```python
from build123d import *

# Parameters (mm, degrees)
BOSS_EXTRUDE1_DEPTH = 5
SKETCH3_R           = 1.25
CUT_EXTRUDE1_DEPTH  = 215.675530355
CIRPATTERN2_COUNT   = 6
FILLET3_R           = 2.5
FILLET4_R           = 60


with BuildPart() as part:
    # Sketch1 → Boss-Extrude1 (new body)
    with BuildSketch(Plane(origin=(0, 0, 0), x_dir=(1, 0, 0), z_dir=(0, 1, 0))):
        Polygon((-81.117712821, 140.5), (-162.235425642, 0), (-81.117712821, -140.5), (81.117712821, -140.5), (162.235425642, 0), (81.117712821, 140.5), align=None)
    extrude(amount=BOSS_EXTRUDE1_DEPTH)

    # Sketch3 → Cut-Extrude1 (cut, through all)
    with BuildSketch(Plane(origin=(0, 5, 0), x_dir=(1, 0, 0), z_dir=(0, 1, 0))):
        with Locations(Location((8.3, 137.1, 0), (0, 0, 270))):
            Circle(SKETCH3_R)
        with Locations(Location((-8.3, 137.1, 0), (0, 0, 270))):
            Circle(SKETCH3_R)
        Polygon((11.75, 140.5), (20.012731221, 109.663067273), (84.964636505, 72.163067273), (115.801569232, 80.425798494), (81.117712821, 140.5), align=None)
    cut_extrude1 = extrude(amount=-CUT_EXTRUDE1_DEPTH, mode=Mode.SUBTRACT)

    # CirPattern2: Cut-Extrude1 ×6 about axis
    cirpattern2_axis = Axis((0, 0, 0), (0, 1, 0))
    for i in range(1, CIRPATTERN2_COUNT):
        add(cut_extrude1.rotate(cirpattern2_axis, i * 360 / CIRPATTERN2_COUNT), mode=Mode.SUBTRACT)

    # Fillet3
    fillet3_edges = [part.edges().sort_by_distance(p)[0] for p in [
        (115.801569232, 2.5, 80.425798494),
        (11.75, 2.5, 140.5),
        (127.551569232, 2.5, -60.074201506),
        (127.551569232, 2.5, 60.074201506),
        (11.75, 2.5, -140.5),
        (115.801569232, 2.5, -80.425798494),
        (-115.801569232, 2.5, -80.425798494),
        (-11.75, 2.5, -140.5),
        (-127.551569232, 2.5, 60.074201506),
        (-127.551569232, 2.5, -60.074201506),
        (-11.75, 2.5, 140.5),
        (-115.801569232, 2.5, 80.425798494),
    ]]
    fillet(fillet3_edges, radius=FILLET3_R)

    # Fillet4
    fillet4_edges = [part.edges().sort_by_distance(p)[0] for p in [
        (20.012731221, 2.5, 109.663067273),
        (84.964636505, 2.5, 72.163067273),
        (104.977367726, 2.5, 37.5),
        (104.977367726, 2.5, -37.5),
        (84.964636505, 2.5, -72.163067273),
        (20.012731221, 2.5, -109.663067273),
        (-20.012731221, 2.5, -109.663067273),
        (-84.964636505, 2.5, -72.163067273),
        (-104.977367726, 2.5, -37.5),
        (-104.977367726, 2.5, 37.5),
        (-84.964636505, 2.5, 72.163067273),
        (-20.012731221, 2.5, 109.663067273),
    ]]
    fillet(fillet4_edges, radius=FILLET4_R)


solid = part.part
```
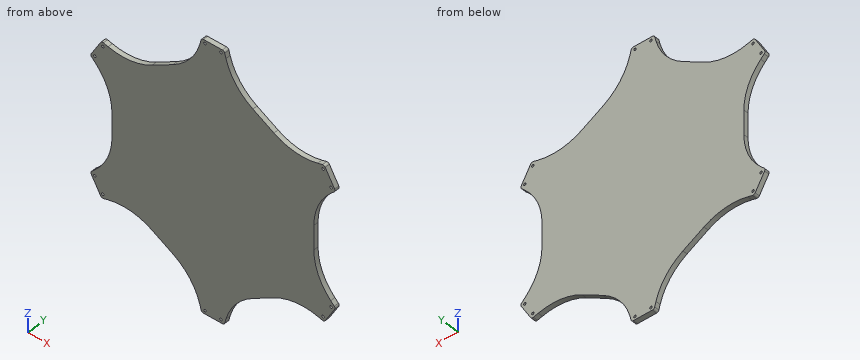
Geometry check sheet. Reference: the model listing, model coordinates, mm. Round coordinates to 2 decimals unless told otherwise and drop trailing zeros. Order: outer loops, then holes, each group sorted by start corner. A loop starts at its lowest first (then second) coordinate and runs counter-clockwise, first axis right, second up. Notation, with made-up numbers: (64, 50) -> (70, 50) arc R15 ccw to (70, 66) -> close; hole circle Ø7 at (89.5, 87.5). An arc over 180 degrees is marked (long way). Return JSON: item names as keys, results as strings. Group by question number.
Q1. Section check B-B, the plane z = -116. Record the boundary of the cut face in (x, y), plus the area to 3 significant figures.
Q2. Material ranges on probe 1 along X at (y, z) = (3.35, -137.1); probe 2 along X at (y, z) = (2.4, -4); probe 3 along Z at (x, y) = (-17, 3.1), recorded low to high. Write a range as from..to.
Q3. Section check A-A, the plane x = -57. Record the boundary of the cut face in (y, z), plus the area to 3 significant figures.
Q4. Gauge pin test, flat ends, axial feed: pin 1 (1.5 mm diameter, centred on x = 18, z = -45, fed in from -Y); pin 2 (2 mm diameter, centred on x = 8.3, z = 137.1, fed in from +Y); pin 3 (1.5 mm diameter, centred on y = 1.5, z = -2.5, fed in from -X); pin 4 (1 mm diameter, centred on y = 1, z = -51.5, fed in from -X). Record the tip position at first contact, or that the pin passes through.
Q5. Section check C-C, the plane y = 3.55. Count the separate pieces of the cut face and the enclosed holes in it, plus the area to 3 significant figures.
Numbers:
{
 "1": {"outline": "(-21.56, 0) -> (21.56, 0) -> (21.56, 5) -> (-21.56, 5) -> close", "area": "216 mm^2"},
 "2": {"probe 1": "-12.66..-9.55, -7.05..7.05, 9.55..12.66", "probe 2": "-104.98..104.98", "probe 3": "-124.18..124.18"},
 "3": {"outline": "(0, -88.31) -> (5, -88.31) -> (5, 88.31) -> (0, 88.31) -> close", "area": "883 mm^2"},
 "4": {"pin 1": "y = 0", "pin 2": "through", "pin 3": "x = -104.98", "pin 4": "x = -119.69"},
 "5": {"separate pieces": "1", "enclosed holes": "12", "area": "43,500 mm^2"}
}
